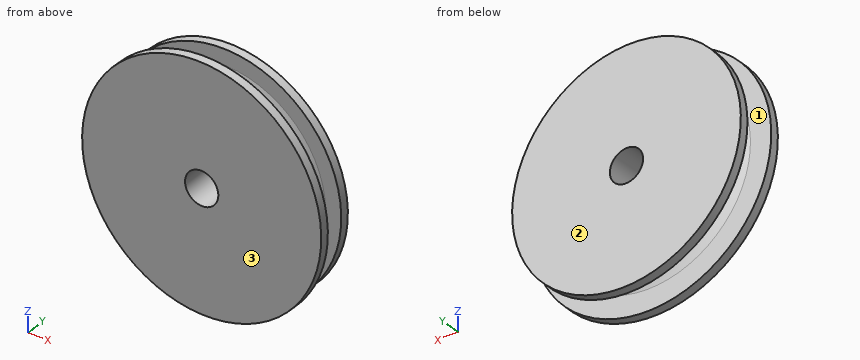
from build123d import *

# Parameters (mm, degrees)
SKETCH1_R           = 9.5
BOSS_EXTRUDE1_DEPTH = 4
SKETCH3_R           = 1.6
CUT_EXTRUDE1_DEPTH  = 15.017845904
SKETCH4_R           = 11
SKETCH4_R_2         = 1.6
EXTENSION_TOP_DEPTH = 0.832825
BOSS_EXTRUDE4_START = -0.832825
SKETCH5_R           = 11.5
SKETCH5_R_2         = 1.6
BOSS_EXTRUDE4_DEPTH = 0.832825


with BuildPart() as part:
    # Sketch1 → Boss-Extrude1 (new body)
    with BuildSketch(Plane(origin=(0, 0, 0), x_dir=(1, 0, 0), z_dir=(0, 1, 0))):
        with Locations(Location((0, 0, 0), (0, 0, 270))):
            Circle(SKETCH1_R)
    extrude(amount=BOSS_EXTRUDE1_DEPTH)

    # Sketch2 → Cut-Revolve3 (revolve, cut)
    with BuildSketch(Plane.XY, mode=Mode.PRIVATE) as cut_revolve3_sk:
        with BuildLine():
            Line((-9.5, 3.167174781), (-9.5, 0.832825219))
            add(Edge.make_bspline(
                [(-9.5, 0.832825219), (-8.911003923, 1.01519245), (-7.940181452, 1.15692307), (-8, 2)],
                knots=[0, 0, 0, 0, 1, 1, 1, 1], degree=3))
            add(Edge.make_bspline(
                [(-9.5, 3.167174781), (-8.911003923, 2.98480755), (-7.940181452, 2.84307693), (-8, 2)],
                knots=[0, 0, 0, 0, 1, 1, 1, 1], degree=3))
        make_face()
    revolve(cut_revolve3_sk.sketch.rotate(Axis((0, 4.2, 0), (0, -1, 0)), 270), axis=Axis((0, 4.2, 0), (0, -1, 0)), mode=Mode.SUBTRACT)

    # Sketch3 → Cut-Extrude1 (cut, through all)
    with BuildSketch(Plane(origin=(0, 4, 0), x_dir=(1, 0, 0), z_dir=(0, 1, 0))):
        with Locations(Location((0, 0, 0), (0, 0, 270))):
            Circle(SKETCH3_R)
    extrude(amount=-CUT_EXTRUDE1_DEPTH, mode=Mode.SUBTRACT)

    # Sketch4 → Extension top (add)
    with BuildSketch(Plane(origin=(0, 4, 0), x_dir=(1, 0, 0), z_dir=(0, 1, 0))):
        with Locations(Location((0, 0, 0), (0, 0, 270))):
            Circle(SKETCH4_R)
        with Locations(Location((0, 0, 0), (0, 0, 270))):
            Circle(SKETCH4_R_2, mode=Mode.SUBTRACT)
    extrude(amount=-EXTENSION_TOP_DEPTH)

    # Sketch5 → Boss-Extrude4 (add)
    with BuildSketch(Plane.XZ.offset(BOSS_EXTRUDE4_START)):
        with Locations(Location((0, 0, 0), (0, 0, 270))):
            Circle(SKETCH5_R)
        with Locations(Location((0, 0, 0), (0, 0, 90))):
            Circle(SKETCH5_R_2, mode=Mode.SUBTRACT)
    extrude(amount=BOSS_EXTRUDE4_DEPTH)


solid = part.part
For this review, take the finished solid that the model builds, in its own axes (mm). Face numbers are marked on the shaded views. Coordinates: 2 decimals unless noted, no trailing zeros. Write each question's results on one line, items separated by ' | '.
Q1. For pin 1 Ø1 at (x, y) = (-1.5, 3.5) entering from +Z; pin 2 Ø2 at (y, z) = (3.5, 9) entering from -X; pin 3 Ø1.5 at (x, y) = (-9, 3.5) entering from +Z; pin 4 Ø2.5 at (x, z) = (0, 0) entering from -Y, all flat-tipped, find the tip position at first contact; note any pin that passes through.
Taken from the geometry:
pin 1: z = 10.95 | pin 2: x = -7.55 | pin 3: z = 7.28 | pin 4: through
Q2. Mouldability with a two-part tool opening along Y and no side actions: class the marked faces 1, 2 and 3 as +Y half, -Y half, draft (parallel to the pull), parting line (faces both ways), or undercut.
Taken from the geometry:
face 1: undercut | face 2: +Y half | face 3: -Y half
Q3. To check wall thickness, follow line 1 along Y through (x, z) = (9.5, -4.25); line 2 along Y through (x, z) = (-8.5, 2.5); line 3 along Z through (x, y) = (0.75, 0.65). State the ranges of each line that lie inside material, in increasing order. Write a range as [from, to].
Taken from the geometry:
line 1: [0, 0.83], [3.17, 4] | line 2: [0, 1.02], [2.98, 4] | line 3: [-11.48, -1.41], [1.41, 11.48]
